from build123d import *

# Parameters (mm, degrees)
BASE_EXTRUSION_DEPTH    = 25.5
ESQUISSE2_W             = 56.002380091
ESQUISSE2_H             = 22.364539332
ENL_V_MAT_EXTRU_1_DEPTH = 79.474518157
ESQUISSE3_W             = 40.935077574
ESQUISSE3_H             = 9.5
ENL_V_MAT_EXTRU_2_DEPTH = 79.474518157
ESQUISSE4_R             = 5
ENL_V_MAT_EXTRU_3_DEPTH = 6
ESQUISSE5_R             = 2.75
ENL_V_MAT_EXTRU_4_DEPTH = 6


with BuildPart() as part:
    # Esquisse1 → Base-Extrusion (new body)
    with BuildSketch(Plane.XY):
        with BuildLine():
            Line((0, 0), (0, 10))
            Line((0, 10), (60, 10))
            Line((60, 10), (72, 3.07179677))
            Line((72, 3.07179677), (72, -8))
            Line((72, -8), (70, -8))
            Line((70, -8), (61, 1))
            Line((61, 1), (52, -8))
            Line((52, -8), (50, -8))
            ThreePointArc((50, -8), (46.526596349, -2.254033308), (40.202041029, 0))
            Line((40.202041029, 0), (0, 0))
        make_face()
    extrude(amount=BASE_EXTRUSION_DEPTH)

    # Esquisse2 → Enlèv. mat.-Extru.1 (cut, through all)
    with BuildSketch(Plane(origin=(0, 10, 0), x_dir=(-1, 0, 0), z_dir=(0, 1, 0))):
        with Locations((-66.001190046, -0.182269666)):
            Rectangle(ESQUISSE2_W, ESQUISSE2_H)
    extrude(amount=-ENL_V_MAT_EXTRU_1_DEPTH, mode=Mode.SUBTRACT)

    # Esquisse3 → Enlèv. mat.-Extru.2 (cut, through all)
    with BuildSketch(Plane(origin=(0, 10, 0), x_dir=(-1, 0, 0), z_dir=(0, 1, 0))):
        with Locations((-58.467538787, 18.25)):
            Rectangle(ESQUISSE3_W, ESQUISSE3_H)
    extrude(amount=-ENL_V_MAT_EXTRU_2_DEPTH, mode=Mode.SUBTRACT)

    # Esquisse4 → Enlèv. mat.-Extru.3 (cut)
    with BuildSketch(Plane.XZ):
        with Locations(Location((10, 5.5, 0), (0, 0, 270))):
            Circle(ESQUISSE4_R)
        with Locations(Location((28, 5.5, 0), (0, 0, 270))):
            Circle(ESQUISSE4_R)
    extrude(amount=-ENL_V_MAT_EXTRU_3_DEPTH, mode=Mode.SUBTRACT)

    # Esquisse5 → Enlèv. mat.-Extru.4 (cut)
    with BuildSketch(Plane.XZ.offset(-6)):
        with Locations(Location((28, 5.5, 0), (0, 0, 270))):
            Circle(ESQUISSE5_R)
        with Locations(Location((10, 5.5, 0), (0, 0, 270))):
            Circle(ESQUISSE5_R)
    extrude(amount=-ENL_V_MAT_EXTRU_4_DEPTH, mode=Mode.SUBTRACT)


solid = part.part
Can you work these out from the model? Positions are in its coordinate system, mm. A direction names the side the tool comes from. Coordinates: 2 decimals unless noted, no trailing zeros. Write each loop counter-clockwise with the first axis right and the second up, starting at its lowest first coordinate (ties: lowest second). Pieces come first, ordered by that corner, then holes.
Q1. Please list where these lines run through material, in increasing order: L1, parallel to X at y = 2.85, z = 5.5; L2, parallel to X at y = 6.8, z = 5.5; L3, parallel to Z at x = 55, y = -4.5.
Results found:
L1: x = 0 to 5, 15 to 23, 33 to 38
L2: x = 0 to 7.25, 12.75 to 25.25, 30.75 to 38
L3: z = 11 to 13.5, 23 to 25.5
Q2. Which directions (+Z, -Z, +X, -X, +Y, -Y) give clear straight access to the entire face, cutting with the end or side of a thin tool? Please do faces 5 (the face through (66, -4, 24)), 6 (the face through (38, 5, 5)), 7 (the face through (55, 3, 13.5)), 8 (the face through (23.12, 2.96, 6.58)).
Results found:
face 5: +Z, -Z, -Y
face 6: -Z, +X, +Y, -Y
face 7: +X, +Y, -Y
face 8: -Y
Q3. Imagine slicing it at C-C, the plane y = 8. List the corners of the cut face in (x, z) for me.
Results found:
outline: (0, 0) - (38, 0) - (38, 11) - (63.46, 11) - (63.46, 13.5) - (38, 13.5) - (38, 23) - (63.46, 23) - (63.46, 25.5) - (0, 25.5) - close; hole circle Ø5.5 at (10, 5.5); hole circle Ø5.5 at (28, 5.5)
Q4. For P1, Ø8, axis at x = 8, z = 5.5, coming from the -Y side; P2, Ø9, axis at x = 49.5, y = 1, coming from the -Z side; P3, Ø8, axis at y = 2.5, z = 6.5, coming from the +X side, each with a flat end and sliding along its axis, tell me the tip position at first contact or that it passes through.
Results found:
P1: stops at y = 0
P2: stops at z = 11
P3: stops at x = 38
Q5. Imagine slicing it at D-D, the plane x = 17.5. List the corners of the cut face in (y, z) for me.
Results found:
outline: (0, 0) - (10, 0) - (10, 25.5) - (0, 25.5) - close
Q6. Imagine slicing it at A-A, the plane z = 5.5. List the corners of the cut face in (x, y) for me.
Results found:
outline: (0, 0) - (5, 0) - (5, 6) - (7.25, 6) - (7.25, 10) - (0, 10) - close; (12.75, 6) - (15, 6) - (15, 0) - (23, 0) - (23, 6) - (25.25, 6) - (25.25, 10) - (12.75, 10) - close; (30.75, 6) - (33, 6) - (33, 0) - (38, 0) - (38, 10) - (30.75, 10) - close
Q7. If we mould it in two halves opening along Z, with no side actions, what happens to faces 1 (the face through (20, 0, 15)), 2 (the face through (55, 3, 11)), 3 (the face through (26, 6, 3)), 4 (the face through (37, 3, 25.5))? For each: +Z half, -Z half, draft (parallel to the pull), parting line (faces both ways), or undercut.
Results found:
face 1: draft
face 2: -Z half
face 3: undercut
face 4: +Z half
Q8. Imagine slicing it at B-B, the plane x = 10. List the corners of the cut face in (y, z) for me.
Results found:
outline: (0, 0) - (10, 0) - (10, 2.75) - (6, 2.75) - (6, 0.5) - (0, 0.5) - close; (0, 10.5) - (6, 10.5) - (6, 8.25) - (10, 8.25) - (10, 25.5) - (0, 25.5) - close
